Geometry: see drawing. Coordinates: mm, zero at the bounding-box minimum. Coordinates: 2 decimals unless noted, no trailing zeros. Loops run counter-clockwise (first coordinate to the right, second up) from the corner with the lowest first, then second, coordinate; pieces in that order, holes last.
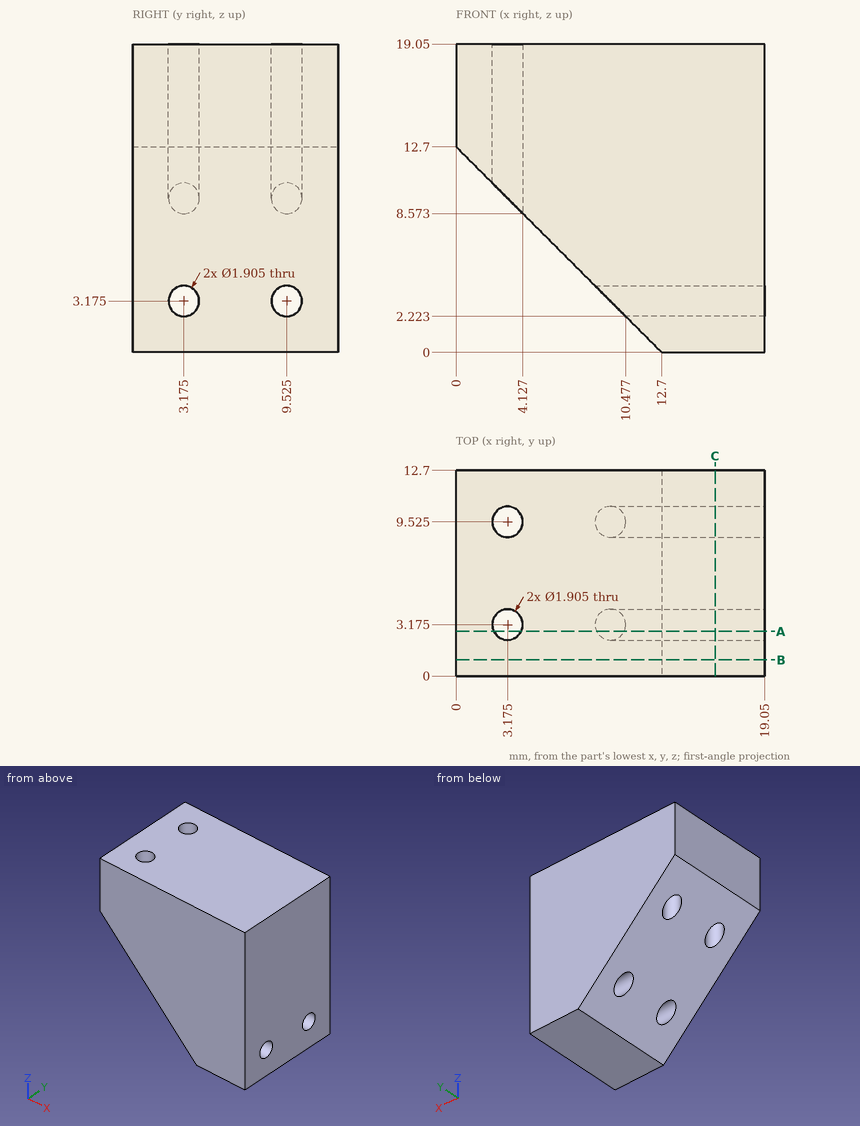
Item 1: Line query: L1, parallel to Y at x = 16.25, z = 3.75 (1 decimal); L2, parallel to Z at x = 2, y = 7; L3, parallel to X at y = 10, z = 9.5. Output: solid intervals per line, ascending.
Result:
L1: y = 0 to 2.4, 3.9 to 8.8, 10.3 to 12.7
L2: z = 10.7 to 19.05
L3: x = 4 to 19.05
Item 2: Section query C-C (x = 16). Count the separate pieces of the cut face and the enclosed holes in it, then the cut area to 3 significant figures.
Result:
separate pieces: 1
enclosed holes: 2
area: 236 mm2
Item 3: Section query B-B (y = 1). Output: boundary loops of the cut face in (x, z).
Result:
outline: (0, 12.7) - (12.7, 0) - (19.05, 0) - (19.05, 19.05) - (0, 19.05) - close
Item 4: Section query A-A (y = 2.75). Output: boundary loops of the cut face in (x, z).
Result:
outline: (0, 12.7) - (2.32, 10.38) - (2.32, 19.05) - (0, 19.05) - close; (4.03, 8.67) - (8.67, 4.03) - (19.05, 4.03) - (19.05, 19.05) - (4.03, 19.05) - close; (10.38, 2.32) - (12.7, 0) - (19.05, 0) - (19.05, 2.32) - close
Item 5: Contact query for flat-ended pins moving along their axis: P1, Ø1.5, axis at x = 5, y = 8.5, coming from the -Z side; P2, Ø1, axis at y = 1.5, z = 11.5, coming from the -X side; P3, Ø2, axis at x = 3.175, y = 3.175, coming from the -Z side (1 decimal); P4, Ø5, axis at x = 14, y = 5, coming from the -Z side. Output: stop coordinate, or through.
Result:
P1: stops at z = 6.95
P2: stops at x = 0.7
P3: stops at z = 8.5
P4: stops at z = 0
